from build123d import *

# Parameters (mm, degrees)
Y_KSEKLIK_EKSTR_ZYON2_DEPTH = 30
KES_EKSTR_ZYON1_REACH       = 62
KES_EKSTR_ZYON2_REACH       = 62
RADYUS1_R                   = 2


with BuildPart() as part:
    # Çizim2 → Yükseklik-Ekstrüzyon2 (new body, symmetric)
    with BuildSketch(Plane(origin=(0, 0, 0), x_dir=(1, 0, 0), z_dir=(0, 1, 0))):
        Polygon((0, 30), (0, -30), (-150, -30), (-150, -21.435935394), (-70, 0), (-150, 21.435935394), (-150, 30), align=None)
    extrude(amount=Y_KSEKLIK_EKSTR_ZYON2_DEPTH, both=True)

    # Çizim3 → Kes-Ekstrüzyon1 (cut, up to next)
    with BuildSketch(Plane.XY.offset(30), mode=Mode.PRIVATE) as kes_ekstr_zyon1_sk1:
        with BuildLine():
            Line((-150, -30), (-30, -30))
            ThreePointArc((-30, -30), (-90, -10), (-150, -30))
        make_face()
    kes_ekstr_zyon1_tool1 = extrude(kes_ekstr_zyon1_sk1.sketch, amount=-KES_EKSTR_ZYON1_REACH, mode=Mode.PRIVATE) & part.part
    add(kes_ekstr_zyon1_tool1.solids().sort_by_distance((-90, -21.927203, 30))[0], mode=Mode.SUBTRACT)

    # Çizim5 → Döndür1 (revolve)
    with BuildSketch(Plane.XY):
        with BuildLine():
            Line((20, -30), (35, -30))
            ThreePointArc((35, -30), (38.535533906, -28.535533906), (40, -25))
            Line((40, -25), (40, -5))
            Line((40, -5), (0, -5))
            Line((0, -5), (0, -20))
            Line((0, -20), (20, -20))
            Line((20, -20), (20, -30))
        make_face()
    revolve(axis=Axis((0, -5, 0), (1, 0, 0)))

    # Çizim6 → Kes-Ekstrüzyon2 (cut, up to next)
    with BuildSketch(Plane.XY.offset(30), mode=Mode.PRIVATE) as kes_ekstr_zyon2_sk1:
        with BuildLine():
            Line((-150, -9.617957362), (-150, 30))
            Line((-150, 30), (0, 30))
            Line((0, 30), (0, 20))
            ThreePointArc((0, 20), (-79.056941504, 25.737381697), (-150, -9.617957362))
        make_face()
    kes_ekstr_zyon2_tool1 = extrude(kes_ekstr_zyon2_sk1.sketch, amount=-KES_EKSTR_ZYON2_REACH, mode=Mode.PRIVATE) & part.part
    add(kes_ekstr_zyon2_tool1.solids().sort_by_distance((-108.440185, 19.830355, 30))[0], mode=Mode.SUBTRACT)

    # Radyus1
    radyus1_edges = [part.edges().sort_by_distance(p)[0] for p in [
        (0, 20, 0),
    ]]
    fillet(radyus1_edges, radius=RADYUS1_R)


solid = part.part
Check sheet for the modelled part. Datum: model origin and axes. Units: mm. A direction names the side the tool comes from. Round coordinates to 2 decimals unless told otherwise and drop trailing zeros. Order: outer loops, then holes, each group sorted by start corner. A loop starts at its lowest first (then second) coordinate and runs counter-clockwise, first axis right, second up.
(1) Access from +Z, -Z, +X, -X, +Y, -Y to the whole of each face (thin tool, end or side, straight path). Record for faces 1 (the flat face through (40, -5, 0)), 2 (the cylindrical face through (27.605, -28.846, -7.509)), 3 (the flat face through (20, 6, 11)).
(2) Scan lines: probe 1 along Z at (x, y) = (-133, 1); probe 2 along Z at (x, y) = (-128, 2.5); probe 3 along Y at (x, z) = (-73.5, 19). Record each from-to range of solid material in increasing order.
(3) Cross-section at A-A, the plane x = -110. Enter the section's corners in (y, z), and give its area (3 significant figures).
(4) Go/stop test with flat-tipped pins: P1, Ø4, axis at y = -2.5, z = -21, coming from the -X side; P2, Ø1, axis at x = -116.5, y = -14.5, coming from the +Z side; P3, Ø5, axis at y = 4, z = -17, coming from the -X side; P4, Ø1, axis at x = -121, z = 16.5, coming from the +Y side. Record where each tip stops, or that it passes through.
(5) Cross-section at B-B, the plane y = -5. Enter the section's corners in (x, z).
(6) Cross-section at D-D, the plane x = -38. Enter the section's corners in (y, z), and give its area (3 significant figures).
(7) Draft check along X on faces 4 (the flat face through (-57, 0, 30)), 5 (the flat face through (0, 11, 0)), 6 (the flat face through (-150, -20, 26)). Enter one of: pulls with the +X half, pulls with the -X half, needs draft (parallel to the pull), parting line crosses it, or undercut.
(8) Cross-section at C-C, the plane y = 25.5. Enter the section's corners in (x, z), and give its area (3 significant figures).
Check sheet entries:
1. face 1: +Z, -Z, +X, +Y, -Y
1. face 2: +X
1. face 3: none
2. probe 1: z = -30 to -16.88, 16.88 to 30
2. probe 2: z = -30 to -15.54, 15.54 to 30
2. probe 3: y = -11.37 to 26.73
3. outline: (-12.02, -30) - (16.06, -30) - (16.06, -10.72) - (-12.02, -10.72) - close; (-12.02, 10.72) - (16.06, 10.72) - (16.06, 30) - (-12.02, 30) - close
3. area: 1,080 mm2
4. P1: stops at x = -143.96
4. P2: passes through
4. P3: stops at x = -135.85
4. P4: stops at y = 10.98
5. outline: (-144.58, -30) - (0, -30) - (0, -15) - (20, -15) - (20, -25) - (35, -25) arc R5 ccw to (40, -20) - (40, 20) arc R5 ccw to (35, 25) - (20, 25) - (20, 15) - (0, 15) - (0, 30) - (-144.58, 30) - (-144.58, 19.98) - (-70, 0) - (-144.58, -19.98) - close
6. outline: (-24.58, -30) - (28.1, -30) - (28.1, 30) - (-24.58, 30) - close
6. area: 3,160 mm2
7. face 4: needs draft
7. face 5: undercut
7. face 6: pulls with the -X half
8. outline: (-80.23, -30) - (-19.77, -30) - (-19.77, 30) - (-80.23, 30) - (-80.23, 2.74) - (-70, 0) - (-80.23, -2.74) - close
8. area: 3,600 mm2
